```python
from build123d import *

# Parameters (mm, degrees)
BOSS_EXTRUDE1_DEPTH = 3.175


with BuildPart() as part:
    # Sketch1 → Boss-Extrude1 (new body)
    with BuildSketch(Plane(origin=(0, 0, 0), x_dir=(1, 0, 0), z_dir=(0, 1, 0))):
        with BuildLine():
            Line((36.786206897, 0), (18.953245729, 0))
            Line((18.953245729, 0), (18.953245729, 3))
            Line((18.953245729, 3), (-6.446754271, 3))
            Line((-6.446754271, 3), (-6.446754271, 0))
            Line((-6.446754271, 0), (-26.713793103, 0))
            add(Edge.make_bspline(
                [(27.346845479, -88.9), (-21.534982329, -59.771214116), (-26.713793103, 0)],
                knots=[0, 0, 0, 1, 1, 1], degree=2))
            Line((27.346845479, -88.9), (36.786206897, -88.9))
            Line((36.786206897, -88.9), (36.786206897, 0))
        make_face()
    extrude(amount=-BOSS_EXTRUDE1_DEPTH)


solid = part.part
```
Here's how the part is built. I have some questions about the finished solid (model axes, mm). A direction names the side the tool comes from. Coordinates: 2 decimals unless noted, no trailing zeros. One line per question, with ' | ' between items.
(1) For faces 1 (the flat face through (12, 0, 32)), 2 (the flat face through (18.953, -2, -1)), 3 (the flat face through (-16, -2, 0)), which set-ups out of +Z, -Z, +X, -X, +Y, -Y let a thin tool reach every point of the face, with its end or its side?
Report:
face 1: +Z, -Z, +X, -X, +Y | face 2: -Z, +X, +Y, -Y | face 3: -Z, -X, +Y, -Y
(2) If I drill on L1, parallel to Z at x = 29.5, y = -1.35; L2, parallel to X at y = -1.7, z = 29.5; L3, parallel to X at y = -2.35, z = 8, over which ranges is the centre line in solid material (lowest first)?
Report:
L1: z = 0 to 88.9 | L2: x = -20.91 to 36.79 | L3: x = -25.81 to 36.79
(3) Will these pins go through, and if not, where does the flat tip stop? pin 1 (1 mm diameter, centred on x = -13, y = -1.5, fed in from +Z); pin 2 (1.5 mm diameter, centred on y = -2.5, z = -1.5, fed in from -X); pin 3 (0.9 mm diameter, centred on y = -1.5, z = -2, fed in from +X).
Report:
pin 1: stops at z = 48.87 | pin 2: stops at x = -6.45 | pin 3: stops at x = 18.95
